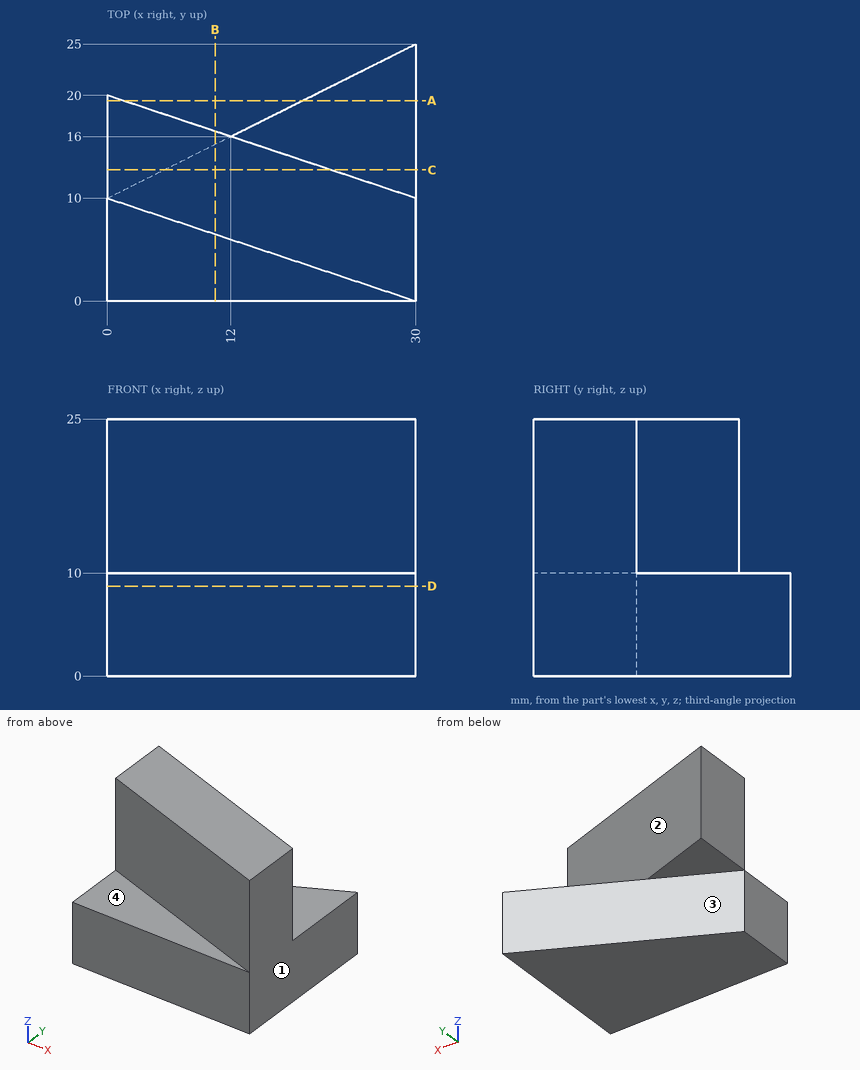
Input: dimensioned drawing with shaded views. Units: mm. Origin: part minimum x, y, z. A direction names the side the tool comes from. Give positions to 0.01 mm unless a question says otherwise; leave off trailing zeros. Loops run counter-clockwise (first coordinate to the right, second up) from the corner with the lowest first, then second, coordinate; pieces in that order, holes last. Notation, with made-up numbers: (11.25, 7.5) -> (56.25, 7.5) arc R17 ccw to (56.25, 26.5) -> close; hole circle Ø1 at (-34.75, 77.5). An arc over 180 degrees is marked (long way). Use a Markdown table: item, result. Add a question column.
1) Line query: line 1 along Z through (x, y) = (14, 16.25); line 2 along X through (y, z) = (15, 2); line 3 along Y through (x, z) = (19.5, 6.5). Output: solid intervals per line, ascending. Write a range as [from, to].
2) Reachability of the marked faces 1, 2, 3 and 4 from +Z, -Z, +X, -X, +Y, -Y: full face, straight path, thin tool, end or side. Return the list, or none.
3) Section query A-A, the plane y = 19.5. Return the cut outline in (x, z).
4) Section query C-C, the plane y = 12.75. Return the cut outline in (x, z), then the cut area to 3 significant figures.
5) Section query B-B, the plane x = 10.5. Return the cut outline in (y, z), then the cut area to 4 significant figures.
6) First-contact query: pin 1 (3 mm diameter, centred on x = 10.5, z = 12.5, fed in from -Y); pin 2 (4.5 mm diameter, centred on x = 23, y = 16, fed in from +Z); pin 3 (10 mm diameter, centred on x = 11.5, z = 17, fed in from +Y). Flat tips, straight axial feed; report the tip coordinate or a pass-through.
7) Section query D-D, the plane z = 8.75. Return the cut outline in (x, y), then the cut area to 3 significant figures.
Numbers:
| question | item | result |
|---|---|---|
| 1 | line 1 | z = [0, 10] |
| 1 | line 2 | x = [10, 30] |
| 1 | line 3 | y = [0, 19.75] |
| 2 | face 1 | +Z, -Z, +X, +Y, -Y |
| 2 | face 2 | +Z, +X, +Y |
| 2 | face 3 | -Z, -X, +Y |
| 2 | face 4 | +Z, -X, -Y |
| 3 | outline | (0, 10) -> (1.5, 10) -> (1.5, 25) -> (0, 25) -> close; (19, 0) -> (30, 0) -> (30, 10) -> (19, 10) -> close |
| 4 | outline | (0, 10) -> (5.5, 10) -> (5.5, 0) -> (30, 0) -> (30, 10) -> (21.75, 10) -> (21.75, 25) -> (0, 25) -> close |
| 4 | area | 571 mm2 |
| 5 | outline | (0, 0) -> (15.25, 0) -> (15.25, 10) -> (16.5, 10) -> (16.5, 25) -> (6.5, 25) -> (6.5, 10) -> (0, 10) -> close |
| 5 | area | 302.5 mm2 |
| 6 | pin 1 | stops at y = 6 |
| 6 | pin 2 | stops at z = 10 |
| 6 | pin 3 | stops at y = 17.83 |
| 7 | outline | (0, 0) -> (30, 0) -> (30, 25) -> (0, 10) -> close |
| 7 | area | 525 mm2 |
